Print and shaded views of the part. All mm, measured from the part's lowest x, y and z. Give positions to 0.01 mm unless a question says otherwise; leave off trailing zeros. Write each loop counter-clockwise with the first axis right and the second up, starting at its lowest first coordinate (ties: lowest second). Pieces come first, ordered by that corner, then holes.
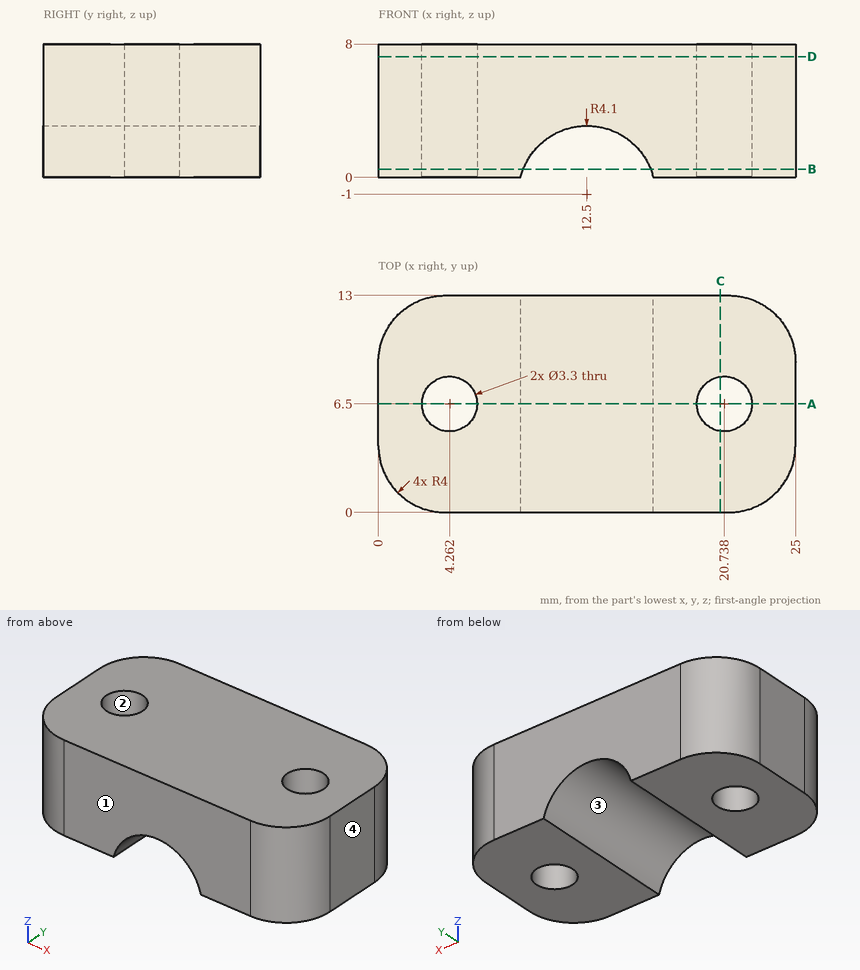
1. Drill centre lines: line 1 along X through (y, z) = (7, 1); line 2 along X through (y, z) = (4.75, 2.75); line 3 along Y through (x, z) = (21.25, 3). Where is each one in solid material? Low to high.
2. Saw through at A-A on y = 6.5. Give the cut face in (x, z).
3. Saw through at D-D on z = 7.25. Give the cut face in (x, y).
4. Saw through at B-B on z = 0.5. Give the cut face in (x, y).
5. Mould opens along X. For the marked faces 1, 2, 3 and 4 say: pulls with the +X half, pulls with the -X half, needs draft (parallel to the pull), parting line crosses it, or undercut.
6. Saw through at C-C on x = 20.5. Give the cut face in (y, z).
7. Drop flat-ended pins along their axis: pin 1 (5 mm diameter, centred on x = 12, y = 2.5, fed in from -Z) (1 decimal); pin 2 (2 mm diameter, centred on x = 4.26, y = 6.5, fed in from +Z). Give the stop position or say it passes through.
Outcome:
1. line 1: x = 0 to 2.69, 5.83 to 8.92, 16.08 to 19.17, 22.31 to 25
1. line 2: x = 0 to 10.84, 14.16 to 25
1. line 3: y = 0.01 to 4.93, 8.07 to 12.99
2. outline: (0, 0) - (2.61, 0) - (2.61, 8) - (0, 8) - close; (5.91, 0) - (8.52, 0) arc R4.1 cw to (16.48, 0) - (19.09, 0) - (19.09, 8) - (5.91, 8) - close; (22.39, 0) - (25, 0) - (25, 8) - (22.39, 8) - close
3. outline: (0, 4) arc R4 ccw to (4, 0) - (21, 0) arc R4 ccw to (25, 4) - (25, 9) arc R4 ccw to (21, 13) - (4, 13) arc R4 ccw to (0, 9) - close; hole circle Ø3.3 at (4.26, 6.5); hole circle Ø3.3 at (20.74, 6.5)
4. outline: (0, 4) arc R4 ccw to (4, 0) - (8.68, 0) - (8.68, 13) - (4, 13) arc R4 ccw to (0, 9) - close; (16.32, 0) - (21, 0) arc R4 ccw to (25, 4) - (25, 9) arc R4 ccw to (21, 13) - (16.32, 13) - close; hole circle Ø3.3 at (4.26, 6.5); hole circle Ø3.3 at (20.74, 6.5)
5. face 1: needs draft
5. face 2: undercut
5. face 3: undercut
5. face 4: pulls with the +X half
6. outline: (0, 0) - (4.87, 0) - (4.87, 8) - (0, 8) - close; (8.13, 0) - (13, 0) - (13, 8) - (8.13, 8) - close
7. pin 1: stops at z = 1.8
7. pin 2: passes through
